Design review of the part built by this model. Coordinates are the model's own, in mm. Face numbers are marked on the shaded views. A direction names the side the tool comes from. Coordinates: 2 decimals unless noted, no trailing zeros. Write each loop counter-clockwise with the first axis right and the second up, starting at its lowest first coordinate (ties: lowest second). Pieces come first, ordered by that corner, then holes.
```python
from build123d import *

# Parameters (mm, degrees)
SKETCH_1_R          = 2.75
SKETCH_1_R_2        = 6.5
EXTRUDE_1_DEPTH     = 10
SKETCH_2_R          = 4.75
CUT_EXTRUDE_2_DEPTH = 6
SKETCH_3_R          = 4.75
CUT_EXTRUDE_3_DEPTH = 6
CUT_EXTRUDE_4_REACH = 1574.343
SKETCH_4_R          = 2.5


with BuildPart() as part:
    # 草图1 → 拉伸1 (new body)
    with BuildSketch(Plane.XY):
        Polygon((1458.024528538, 1041.679154631), (1458.024528538, 1025.679154631), (1451.024528538, 1025.679154631), (1451.024528538, 1011.679154631), (1566.024528538, 1011.679154631), (1572.024528538, 1017.679154631), (1572.024528538, 1035.679154631), (1566.024528538, 1041.679154631), align=None)
        with Locations((1545.524528538, 1016.679154631)):
            Circle(SKETCH_1_R, mode=Mode.SUBTRACT)
        with Locations((1485.524528538, 1016.679154631)):
            Circle(SKETCH_1_R, mode=Mode.SUBTRACT)
        with Locations((1485.524528538, 1036.679154631)):
            Circle(SKETCH_1_R, mode=Mode.SUBTRACT)
        with Locations((1545.524528538, 1036.679154631)):
            Circle(SKETCH_1_R, mode=Mode.SUBTRACT)
        with Locations((1496.024528538, 1021.179154631)):
            Circle(SKETCH_1_R, mode=Mode.SUBTRACT)
        with Locations((1535.024528538, 1021.179154631)):
            Circle(SKETCH_1_R, mode=Mode.SUBTRACT)
        with Locations((1535.024528538, 1034.679154631)):
            Circle(SKETCH_1_R, mode=Mode.SUBTRACT)
        with Locations((1496.024528538, 1034.679154631)):
            Circle(SKETCH_1_R, mode=Mode.SUBTRACT)
        with Locations((1562.024528538, 1022.679154631)):
            Circle(SKETCH_1_R_2, mode=Mode.SUBTRACT)
        with BuildLine():
            Line((1508.024528538, 1035.679154631), (1523.024528538, 1035.679154631))
            ThreePointArc((1523.024528538, 1035.679154631), (1530.024528538, 1028.679154631), (1523.024528538, 1021.679154631))
            Line((1523.024528538, 1021.679154631), (1508.024528538, 1021.679154631))
            ThreePointArc((1508.024528538, 1021.679154631), (1501.024528538, 1028.679154631), (1508.024528538, 1035.679154631))
        make_face(mode=Mode.SUBTRACT)
    extrude(amount=EXTRUDE_1_DEPTH)

    # 草图2 → 拉伸2 (cut)
    with BuildSketch(Plane.XY.offset(10)):
        with Locations((1485.524528538, 1036.679154631)):
            Circle(SKETCH_2_R)
        with Locations((1545.524528538, 1036.679154631)):
            Circle(SKETCH_2_R)
        with Locations((1485.524528538, 1016.679154631)):
            Circle(SKETCH_2_R)
        with Locations((1545.524528538, 1016.679154631)):
            Circle(SKETCH_2_R)
    extrude(amount=-CUT_EXTRUDE_2_DEPTH, mode=Mode.SUBTRACT)

    # 草图3 → 拉伸3 (cut)
    with BuildSketch(Plane(origin=(0, 0, 0), x_dir=(-1, 0, 0), z_dir=(0, 0, -1))):
        with Locations((-1535.024528538, 1034.679154631)):
            Circle(SKETCH_3_R)
        with Locations((-1496.024528538, 1034.679154631)):
            Circle(SKETCH_3_R)
        with Locations((-1535.024528538, 1021.179154631)):
            Circle(SKETCH_3_R)
        with Locations((-1496.024528538, 1021.179154631)):
            Circle(SKETCH_3_R)
    extrude(amount=-CUT_EXTRUDE_3_DEPTH, mode=Mode.SUBTRACT)

    # 草图4 → 拉伸4 (cut, up to next)
    with BuildSketch(Plane(origin=(0, 1041.679154631, 0), x_dir=(1, 0, 0), z_dir=(0, 1, 0)), mode=Mode.PRIVATE) as cut_extrude_4_sk1:
        with Locations(Location((1505.524528538, -5, 0), (0, 0, 270))):
            Circle(SKETCH_4_R)
    cut_extrude_4_tool1 = extrude(cut_extrude_4_sk1.sketch, amount=-CUT_EXTRUDE_4_REACH, mode=Mode.PRIVATE) & part.part
    # 草图4 → 拉伸4 (cut, up to next)
    with BuildSketch(Plane(origin=(0, 1041.679154631, 0), x_dir=(1, 0, 0), z_dir=(0, 1, 0)), mode=Mode.PRIVATE) as cut_extrude_4_sk2:
        with Locations(Location((1525.524528538, -5, 0), (0, 0, 270))):
            Circle(SKETCH_4_R)
    cut_extrude_4_tool2 = extrude(cut_extrude_4_sk2.sketch, amount=-CUT_EXTRUDE_4_REACH, mode=Mode.PRIVATE) & part.part
    add(cut_extrude_4_tool1.solids().sort_by_distance((1505.524529, 1041.679155, 5))[0], mode=Mode.SUBTRACT)
    add(cut_extrude_4_tool2.solids().sort_by_distance((1525.524529, 1041.679155, 5))[0], mode=Mode.SUBTRACT)


solid = part.part
```
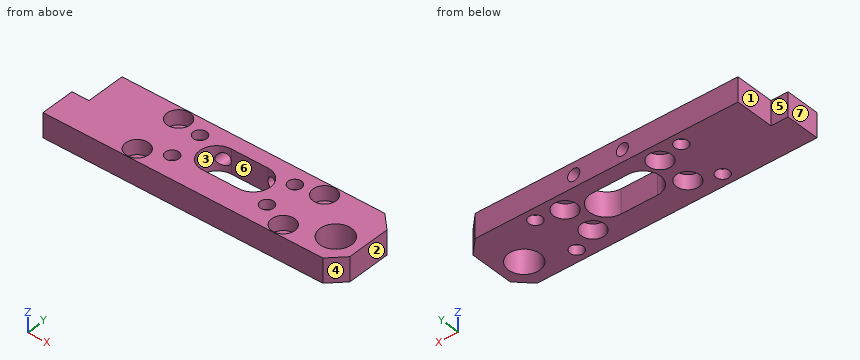
(1) Consider section B-B (x = 1558). Give the boundary of the cut face in (y, z), plus the area to 3 significant figures.
(2) Consider section A-A (x = 1522). Give the boundary of the cut face in (y, z).
(3) Insertion check: pin 1 Ø5 at (y, z) = (1038.5, 8.5) entering from -X; pin 2 Ø6.5 at (x, y) = (1485.52, 1016.68) entering from +Z. Each pin has a flat end and moves straight along its axis. Give the tip position at first contact, or say it passes through.
(4) Mouldability with a two-part tool opening along X and no side actions: class the marked faces 4, 5, 6 and 7 as +X half, -X half, draft (parallel to the pull), parting line (faces both ways), or undercut.
(5) Wall thickness on line 1 (X direction, y = 1040, z = 5); line 2 (Y direction, x = 1536, z = 2); line 3 (X direction, y = 1018, z = 9.25): over which ranges is each line inside the solid? List them lowest first.
(6) For the marked faces 1, 2 and 3, list the 3-axis set-ups (+Z, -Z, +X, -X, +Y, -Y) from which the entire face can be reached by the end or side of a thin tool; tool diameter is ignored.
Results:
1. outline: (1011.68, 0) - (1017.57, 0) - (1017.57, 10) - (1011.68, 10) - close; (1027.78, 0) - (1041.68, 0) - (1041.68, 10) - (1027.78, 10) - close
1. area: 198 mm2
2. outline: (1011.68, 0) - (1021.68, 0) - (1021.68, 10) - (1011.68, 10) - close; (1035.68, 0) - (1041.68, 0) - (1041.68, 10) - (1035.68, 10) - close
3. pin 1: stops at x = 1458.02
3. pin 2: stops at z = 4
4. face 4: +X half
4. face 5: draft
4. face 6: undercut
4. face 7: -X half
5. line 1: x = 1458.02 to 1482.13, 1488.92 to 1503.02, 1508.02 to 1523.02, 1528.02 to 1542.13, 1548.92 to 1567.7
5. line 2: y = 1011.68 to 1016.53, 1025.83 to 1030.03, 1039.33 to 1041.68
5. line 3: x = 1451.02 to 1480.96, 1490.09 to 1540.96, 1550.09 to 1557.51, 1566.54 to 1572.02
6. face 1: +Z, -Z, -X, +Y
6. face 2: +Z, -Z, +X, +Y, -Y
6. face 3: +Z, -Z
